For this review, take the finished solid that the model builds, in its own axes (mm). A direction names the side the tool comes from. Give positions to 0.01 mm unless a question says otherwise; leave off trailing zeros. Loops run counter-clockwise (first coordinate to the right, second up) from the corner with the lowest first, then second, coordinate; pieces in that order, holes last. Notation, with made-up numbers: (77, 24) - (121, 24) arc R12 ccw to (121, 40) - close; hole circle Ø6 at (7.25, 79.25). An arc over 180 degrees is marked (long way). Answer as CSV lines item,"result".
from build123d import *

# Parameters (mm, degrees)
EXTRUDE_1_DEPTH     = 85
EXTRUDE_650_DEPTH   = 440
EXTRUDE_2_DEPTH     = 85
SKETCH_5_R          = 115
CUT_EXTRUDE_1_DEPTH = 693.42779407


with BuildPart() as part:
    # Эскиз2 → Боковой многогранник 1 (new body)
    with BuildSketch(Plane(origin=(0, 0, 0), x_dir=(1, 0, 0), z_dir=(0, 1, 0))):
        Polygon((0, 176.091832103), (-152.5, 88.045916051), (-152.5, -88.045916051), (0, -176.091832103), (152.5, -88.045916051), (152.5, 88.045916051), align=None)
    extrude(amount=EXTRUDE_1_DEPTH)

    # Sketch 292 → Extrude 650 (add)
    with BuildSketch(Plane(origin=(0, 0, 0), x_dir=(1, 0, 0), z_dir=(0, 1, 0))):
        Polygon((0, 161.658075373), (-140, 80.829037687), (-140, -80.829037687), (-47.5, -134.233937587), (-47.5, -195), (-132.5, -195), (-132.5, -290), (132.5, -290), (132.5, -195), (47.5, -195), (47.5, -134.233937587), (140, -80.829037687), (140, 80.829037687), align=None)
    extrude(amount=-EXTRUDE_650_DEPTH)

    # Эскиз4 → Боковой многогранник 2 (add)
    with BuildSketch(Plane.XZ.offset(440)):
        Polygon((0, -176.091832103), (152.5, -88.045916051), (152.5, 88.045916051), (0, 176.091832103), (-152.5, 88.045916051), (-152.5, -88.045916051), align=None)
    extrude(amount=EXTRUDE_2_DEPTH)

    # Эскиз5 → Вырез-Вытянуть1 (cut, through all)
    with BuildSketch(Plane(origin=(0, 85, 0), x_dir=(1, 0, 0), z_dir=(0, 1, 0))):
        with Locations(Location((0, 0, 0), (0, 0, 270))):
            Circle(SKETCH_5_R)
    extrude(amount=-CUT_EXTRUDE_1_DEPTH, mode=Mode.SUBTRACT)


solid = part.part
1) Wall thickness on line 1 (X direction, y = -219, z = 0); line 2 (Z direction, x = -80, y = -110.5); line 3 (X direction, y = -485, z = 74): over which ranges is each line inside the solid? List them lowest first. Write a range as from..to.
From the geometry:
line 1,"x = -140..-115, 115..140"
line 2,"z = -115.47..-82.61, 82.61..115.47, 195..290"
line 3,"x = -152.5..-88.03, 88.03..152.5"
2) Consider section C-C on x = -67. Write out the cut boundary in (y, z).
From the geometry:
outline,"(-525, -137.41) - (-440, -137.41) - (-440, -122.98) - (0, -122.98) - (0, -137.41) - (85, -137.41) - (85, -93.47) - (-525, -93.47) - close; (-525, 93.47) - (85, 93.47) - (85, 137.41) - (0, 137.41) - (0, 122.98) - (-440, 122.98) - (-440, 137.41) - (-525, 137.41) - close; (-440, 195) - (0, 195) - (0, 290) - (-440, 290) - close"
3) Consider section A-A on z = 0. Write out the cut boundary in (x, y), and give its area (4 significant figures).
From the geometry:
outline,"(-152.5, -525) - (-115, -525) - (-115, 85) - (-152.5, 85) - (-152.5, 0) - (-140, 0) - (-140, -440) - (-152.5, -440) - close; (115, -525) - (152.5, -525) - (152.5, -440) - (140, -440) - (140, 0) - (152.5, 0) - (152.5, 85) - (115, 85) - close"
area,"34,750 mm^2"
4) Consider section D-D on y = -483. Write out the cut boundary in (x, z), and give its area (3 significant figures).
From the geometry:
outline,"(-152.5, -88.05) - (0, -176.09) - (152.5, -88.05) - (152.5, 88.05) - (0, 176.09) - (-152.5, 88.05) - close; hole circle Ø230 at (0, 0)"
area,"39,000 mm^2"
5) Machinability: for faces 1 (the flat face through (75.183, 41.905, 132.685)), 2 (the flat face through (-140, -217, -1)), 3 (the flat face through (93.103, -216.92, 107.905)), 4 (the flat face through (-77.32, 41.9, 131.45)), which of the approach directions +Z, -Z, +X, -X, +Y, -Y give a long, thin tool a straight path to every point of the face, cutting with its end or side? Answer none if there is none.
From the geometry:
face 1,"+Z, +X, +Y"
face 2,"+Z, -Z, -X"
face 3,"+X"
face 4,"+Z, -X, +Y"
6) Consider section B-B on y = -422. Write out the cut boundary in (x, z).
From the geometry:
outline,"(-140, -80.83) - (0, -161.66) - (140, -80.83) - (140, 80.83) - (47.5, 134.23) - (47.5, 195) - (132.5, 195) - (132.5, 290) - (-132.5, 290) - (-132.5, 195) - (-47.5, 195) - (-47.5, 134.23) - (-140, 80.83) - close; hole circle Ø230 at (0, 0)"
7) Insertion check: P1, Ø8, axis at y = -78, z = -23.5, coming from the -X side; P2, Ø3, axis at y = -424.5, z = 44.5, coming from the +X side; P3, Ø4, axis at x = -118.5, y = -123.5, coming from the -Z side. Each pin has a flat end and moves straight along its axis. Give the tip position at first contact, or say it passes through.
From the geometry:
P1,"stops at x = -140"
P2,"stops at x = 140"
P3,"stops at z = -94.4"
8) Draft analysis for pull direction Z (two halves, no side actions). For faces 5 (the flat face through (-47.5, -217, 164)), 6 (the flat face through (-2, 0, 234)), 7 (the flat face through (75.183, -481.905, -132.685)), state which applies: pulls with the +Z half, pulls with the -Z half, needs draft (parallel to the pull), parting line crosses it, or undercut.
From the geometry:
face 5,"undercut"
face 6,"needs draft"
face 7,"pulls with the -Z half"
